from build123d import *

# Parameters (mm, degrees)
SKETCH1_R           = 1.5
BOSS_EXTRUDE1_DEPTH = 2


with BuildPart() as part:
    # Sketch1 → Boss-Extrude1 (new body)
    with BuildSketch(Plane(origin=(0, 0, 0), x_dir=(1, 0, 0), z_dir=(0, 1, 0))):
        Polygon((-6, 21.735699927), (-8, 21.735699927), (-8, 26.735699927), (8, 26.735699927), (8, 21.735699927), (6, 21.735699927), (6, -15.764300073), (-6, -15.764300073), align=None)
        with Locations(Location((0, -10.764300073, 0), (0, 0, 270))):
            Circle(SKETCH1_R, mode=Mode.SUBTRACT)
        with BuildLine():
            Line((1.5, 2.735699927), (1.5, 11.735699927))
            ThreePointArc((1.5, 11.735699927), (0, 13.235699927), (-1.5, 11.735699927))
            Line((-1.5, 11.735699927), (-1.5, 2.735699927))
            ThreePointArc((-1.5, 2.735699927), (0, 1.235699927), (1.5, 2.735699927))
        make_face(mode=Mode.SUBTRACT)
    extrude(amount=BOSS_EXTRUDE1_DEPTH)


solid = part.part
The listing builds one solid part. Answer for the finished solid, in the listing's coordinates (mm). A direction names the side the tool comes from. Give positions to 0.01 mm unless a question says otherwise; leave off trailing zeros. Loops run counter-clockwise (first coordinate to the right, second up) from the corner with the lowest first, then second, coordinate; pieces in that order, holes last.
Item 1: A cutting plane is placed at D-D (x = 6.5). Give the vertices of the cut face in (y, z), then the cut area to 3 significant figures.
Derived:
outline: (0, -26.74) - (2, -26.74) - (2, -21.74) - (0, -21.74) - close
area: 10.0 mm2
Item 2: Each of these flat-tipped pins is pushed along its axis until it touches: pin 1 Ø0.6 at (x, y) = (7, 1) entering from +Z; pin 2 Ø0.6 at (y, z) = (1.5, -7.5) entering from -X; pin 3 Ø1 at (y, z) = (1, -10.5) entering from +X; pin 4 Ø4 at (x, z) = (0, 10.76) entering from -Y. Where does it stop, or does it pass through?
Derived:
pin 1: stops at z = -21.74
pin 2: stops at x = -6
pin 3: stops at x = 6
pin 4: stops at y = 0
Item 3: Find the intervals of material crossed by line 1 along X through (y, z) = (1.65, -10); line 2 along Z through (x, y) = (-0.75, 1.95); line 3 along X through (y, z) = (0.95, -19.5), in increasing order.
Derived:
line 1: x = -6 to -1.5, 1.5 to 6
line 2: z = -26.74 to -13.03, -1.44 to 9.47, 12.06 to 15.76
line 3: x = -6 to 6
Item 4: A cutting plane is placed at B-B (x = 0). Give the vertices of the cut face in (y, z).
Derived:
outline: (0, -26.74) - (2, -26.74) - (2, -13.24) - (0, -13.24) - close; (0, -1.24) - (2, -1.24) - (2, 9.26) - (0, 9.26) - close; (0, 12.26) - (2, 12.26) - (2, 15.76) - (0, 15.76) - close
Item 5: A cutting plane is placed at A-A (z = -8). Give the vertices of the cut face in (x, y).
Derived:
outline: (-6, 0) - (-1.5, 0) - (-1.5, 2) - (-6, 2) - close; (1.5, 0) - (6, 0) - (6, 2) - (1.5, 2) - close
Item 6: A cutting plane is placed at C-C (y = 0.95). Give the vertices of the cut face in (x, z), then the cut area to 3 significant figures.
Derived:
outline: (-8, -26.74) - (8, -26.74) - (8, -21.74) - (6, -21.74) - (6, 15.76) - (-6, 15.76) - (-6, -21.74) - (-8, -21.74) - close; hole (-1.5, -11.74) arc R1.5 ccw to (1.5, -11.74) - (1.5, -2.74) arc R1.5 ccw to (-1.5, -2.74) - close; hole circle Ø3 at (0, 10.76)
area: 489 mm2
Item 7: Determine the mould class of faces 4 (the cylindrical face through (-0.033, 0.986, -1.236)), 5 (the flat face through (-7, 1, -21.736)), 6 (the flat face through (-8, 1, -24)) for opening direction Z: +Z half, -Z half, draft (parallel to the pull), parting line (faces both ways), or undercut.
Derived:
face 4: undercut
face 5: +Z half
face 6: draft
Item 8: A tool of negligible diameter and unlimited length cuts with its end or side. For faces 1 (the flat face through (-1.5, 1, -7)), 2 (the flat face through (7, 1, -21.736)), 3 (the flat face through (-6, 1, -3)), from which of +Z, -Z, +X, -X, +Y, -Y can it reach the whole face along a straight path? Write none if from no direction.
Derived:
face 1: +Y, -Y
face 2: +Z, +X, +Y, -Y
face 3: +Z, -X, +Y, -Y
